For this review, take the finished solid that the model builds, in its own axes (mm). A direction names the side the tool comes from. Give positions to 0.01 mm unless a question says otherwise; leave off trailing zeros. Loops run counter-clockwise (first coordinate to the right, second up) from the corner with the lowest first, then second, coordinate; pieces in that order, holes last. Notation, with made-up numbers: (28.25, 21.5) - (67.25, 21.5) arc R19 cw to (67.25, 37.5) - close; hole circle Ø5 at (-5.5, 9). An arc over 180 degrees is marked (long way). Put each result on its own line as item: value.
from build123d import *

# Parameters (mm, degrees)
F0_W     = 127
F0_H     = 76.2
F1_DEPTH = 25.4
F2_W     = 127
F2_H     = 25.4
F3_DEPTH = 127
F5_DEPTH = 25.4
F6_R     = 31.75
F7_DEPTH = 25.401
F8_W     = 25.4
F8_H     = 25.4
F9_DEPTH = 25.401


with BuildPart() as f1:
    # F0 (on Front) → F1 (new body)
    with BuildSketch(Plane.XZ):
        Rectangle(F0_W, F0_H)
    extrude(amount=-F1_DEPTH)

    # F2 (on face) → F3 (join)
    with BuildSketch(Plane.XZ):
        with Locations((0, -25.4)):
            Rectangle(F2_W, F2_H)
    extrude(amount=F3_DEPTH)

    # F4 (on face) → F5 (cut)
    with BuildSketch(Plane.XY.offset(-12.7)):
        with BuildLine():
            Line((-63.5, -127), (0, -127))
            ThreePointArc((0, -127), (-44.901281, -108.401281), (-63.5, -63.5))
            Line((-63.5, -63.5), (-63.5, -127))
        make_face()
        with BuildLine():
            ThreePointArc((63.5, -63.5), (44.901281, -108.401281), (0, -127))
            Line((0, -127), (63.5, -127))
            Line((63.5, -127), (63.5, -63.5))
        make_face()
    extrude(amount=-F5_DEPTH, mode=Mode.SUBTRACT)

    # F6 (on face) → F7 (cut, through all)
    with BuildSketch(Plane.XY.offset(-12.7)):
        with Locations((0, -63.5)):
            Circle(F6_R)
    extrude(amount=-F7_DEPTH, mode=Mode.SUBTRACT)

    # F8 (on face) → F9 (cut, through all)
    with BuildSketch(Plane.XZ):
        with Locations((-50.8, 25.4)):
            Rectangle(F8_W, F8_H)
    extrude(amount=-F9_DEPTH, mode=Mode.SUBTRACT)


solid = f1.part
1) Take a section at C-C on y = 9. State the section outline as (x, z) points, and give its area (3 significant figures).
Geometry check:
outline: (-63.5, -38.1) - (63.5, -38.1) - (63.5, 38.1) - (-38.1, 38.1) - (-38.1, 12.7) - (-63.5, 12.7) - close
area: 9,030 mm²
2) Draft analysis for pull direction X (two halves, no side actions). For faces 4 (the face through (-63.5, -9, -19)), 5 (the face through (63.5, -9, -17)), 6 (the face through (-6.883, -94.495, -25.222)), 7 (the face through (13, -34, -12.7)), state which applies: pulls with the +X half, pulls with the -X half, needs draft (parallel to the pull), parting line crosses it, or undercut.
Geometry check:
face 4: pulls with the -X half
face 5: pulls with the +X half
face 6: undercut
face 7: needs draft
3) Wall thickness on line 1 (Z direction, x = -52, y = -90); line 2 (Y direction, x = 13, z = 6.5); line 3 (Z direction, x = -41, y = 8): over which ranges is each line inside the solid? List them lowest first.
Geometry check:
line 1: z = -38.1 to -12.7
line 2: y = 0 to 25.4
line 3: z = -38.1 to 12.7
4) For faces 1 (the face through (-38.1, 13, 25)), 2 (the face through (12, 13, 38.1)), 3 (the face through (-1, 0, 13)), list the 3-axis set-ups (+Z, -Z, +X, -X, +Y, -Y) from which the entire face can be reached by the end or side of a thin tool; tool diameter is ignored.
Geometry check:
face 1: +Z, -X, +Y, -Y
face 2: +Z, +X, -X, +Y, -Y
face 3: +Z, +X, -X, -Y
5) Insertion check: pin 1 Ø12 at (x, y) = (8.5, -25.5) entering from +Z; pin 2 Ø4 at (x, z) = (30.5, 17) entering from -Y; pin 3 Ø2 at (x, z) = (-21, -25) entering from -Y. Each pin has a flat end and moves straight along its axis. Give the tip position at first contact, or say it passes through.
Geometry check:
pin 1: stops at z = -12.7
pin 2: stops at y = 0
pin 3: stops at y = -123.77
6) Take a section at A-A on z = -27. State the section outline as (x, y) points, and give its area (3 significant figures).
Geometry check:
outline: (-63.5, -63.5) arc R63.5 ccw to (0, -127) arc R63.5 ccw to (63.5, -63.5) - (63.5, 25.4) - (-63.5, 25.4) - close; hole circle Ø63.5 at (0, -63.5)
area: 14,500 mm²
7) Take a section at D-D on x = -25. State the section outline as (y, z) points, and give its area (3 significant figures).
Geometry check:
outline: (-121.87, -38.1) - (-83.07, -38.1) - (-83.07, -12.7) - (-121.87, -12.7) - close; (-43.93, -38.1) - (25.4, -38.1) - (25.4, 38.1) - (0, 38.1) - (0, -12.7) - (-43.93, -12.7) - close
area: 4,040 mm²
8) Take a section at B-B on x = 14.5. State the section outline as (y, z) points.
Geometry check:
outline: (-125.32, -38.1) - (-91.75, -38.1) - (-91.75, -12.7) - (-125.32, -12.7) - close; (-35.25, -38.1) - (25.4, -38.1) - (25.4, 38.1) - (0, 38.1) - (0, -12.7) - (-35.25, -12.7) - close
